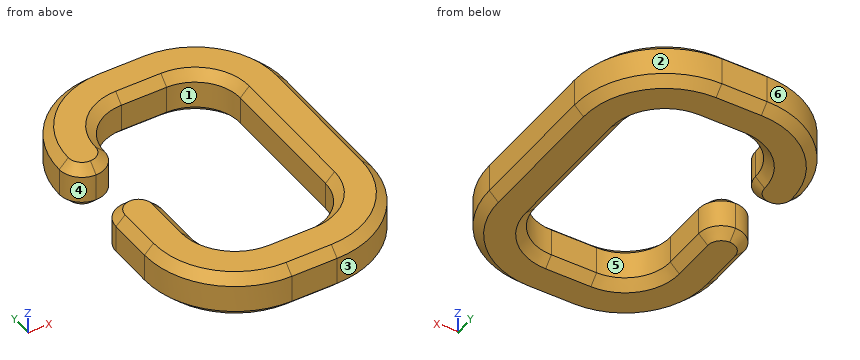
```python
from build123d import *

# Parameters (mm, degrees)
F0_W     = 10
F0_H     = 15
F0_H_2   = 50
F0_H_3   = 25
F1_DEPTH = 10
F2_R     = 10
F3_R     = 20
F4_R     = 4.99999
F5_SIZE  = 2


# Not quite as in the source:
# - a fillet or chamfer is up to 0.001 mm smaller than in the source, because OpenCascade refuses the exact size


with BuildPart() as f1:
    # F0 (on Top) → F1 (new body)
    with BuildSketch(Plane.XY):
        with Locations((-40, 17.5)):
            Rectangle(F0_W, F0_H)
        Polygon((-35, 25), (-5, 25), (5, 25), (5, 35), (-45, 35), (-45, 25), align=None)
        Rectangle(F0_W, F0_H_2)
        Polygon((5, -25), (-5, -25), (-35, -25), (-45, -25), (-45, -35), (5, -35), align=None)
        with Locations((-40, -12.5)):
            Rectangle(F0_W, F0_H_3)
    extrude(amount=F1_DEPTH)

    # F2
    f2_edges = [f1.edges().sort_by_distance(p)[0] for p in [
        (-35, 25, 5),
        (-5, 25, 5),
        (-5, -25, 5),
        (-35, -25, 5),
    ]]
    fillet(f2_edges, radius=F2_R)

    # F3
    f3_edges = [f1.edges().sort_by_distance(p)[0] for p in [
        (5, 35, 5),
        (-45, 35, 5),
        (5, -35, 5),
        (-45, -35, 5),
    ]]
    fillet(f3_edges, radius=F3_R)

    # F4 (radius 5 in the source; OpenCascade refuses exactly that, so slightly less here)
    f4_edges = [f1.edges().sort_by_distance(p)[0] for p in [
        (-35, 10, 5),
        (-45, 10, 5),
        (-45, 0, 5),
        (-35, 0, 5),
    ]]
    fillet(f4_edges, radius=F4_R)

    # F5
    f5_edges = [f1.edges().sort_by_distance(p)[0] for p in [
        (-45, -9.999995, 0),
        (-39.142136, -29.142136, 10),
    ]]
    chamfer(f5_edges, length=F5_SIZE)


solid = f1.part
```
Work out the finished part from the listing and answer in its coordinate system (mm). Face numbers are marked on the shaded views. A direction names the side the tool comes from. Give positions to 0.01 mm unless a question says otherwise; leave off trailing zeros. Loops run counter-clockwise (first coordinate to the right, second up) from the corner with the lowest first, then second, coordinate; pieces in that order, holes last. Notation, with made-up numbers: (-33.5, 33) -> (21.5, 33) arc R14 cw to (21.5, 59) -> close; hole circle Ø7 at (7, 42). An arc over 180 degrees is marked (long way). Put each result on its own line as item: value. Start each with the question number.
Item 1: Each of these flat-tipped pins is pushed along its axis until it touches: P1, Ø5, axis at x = -32.5, z = 4.5, coming from the +Y side; P2, Ø1.8, axis at y = 6.5, z = 4.5, coming from the -X side; P3, Ø8, axis at x = -37.5, y = 4.5, coming from the +Z side. Where does it stop, or does it pass through?
Item 2: Which of the six approach directions +Z, -Z, +X, -X, +Y, -Y give full straight-line access (tool end or side, diameter ignored) to the marked faces 4, 5 and 6?
Item 3: The mould has two halves that part along Y. Classify the marked faces 1, 2 and 3: released by +Y, released by -Y, zero draft, split by the parting line, or undercut.
Item 4: Find the intervals of material crossed by L1, parallel to Y at x = -21, z = 7; L2, parallel to X at y = -15, z = 3.25; L3, parallel to Y at x = 1, z = 2, in increasing order. Write a range as [from, to].
Item 5: The part is cut by section A-A (y = -8.5). Give the vertices of the cut face in (x, z), then the cut area to 3 significant figures.
Item 6: The part is cut by section C-C (y = 2). Give the vertices of the cut face in (x, z), then the cut area to 3 significant figures.
Answers below:
1. P1: y = 34.36
1. P2: x = -5
1. P3: through
2. face 4: +Z, -Z, -X
2. face 5: +Z, -Z
2. face 6: +Z, -Z, -X, +Y
3. face 1: undercut
3. face 2: released by +Y
3. face 3: released by -Y
4. L1: [-35, -25], [25, 35]
4. L2: [-45, -35], [-5, 5]
4. L3: [-27, 27]
5. outline: (-45, 2) -> (-43, 0) -> (-37, 0) -> (-35, 2) -> (-35, 8) -> (-37, 10) -> (-43, 10) -> (-45, 8) -> close; (-5, 2) -> (-3, 0) -> (3, 0) -> (5, 2) -> (5, 8) -> (3, 10) -> (-3, 10) -> (-5, 8) -> close
5. area: 184 mm2
6. outline: (-5, 2) -> (-3, 0) -> (3, 0) -> (5, 2) -> (5, 8) -> (3, 10) -> (-3, 10) -> (-5, 8) -> close
6. area: 92.0 mm2
